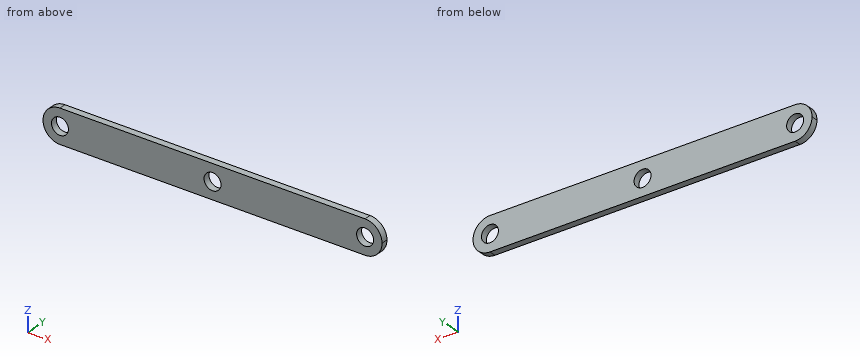
```python
from build123d import *

# Parameters (mm, degrees)
F0_W     = 100
F0_H     = 10
F0_R     = 2.5
F1_DEPTH = 2
F2_R     = 4.99999


# Not quite as in the source:
# - a fillet or chamfer is up to 0.001 mm smaller than in the source, because OpenCascade refuses the exact size


with BuildPart() as f1:
    # F0 (on Front) → F1 (new body)
    with BuildSketch(Plane.XZ):
        Rectangle(F0_W, F0_H)
        with Locations((-45, 0)):
            Circle(F0_R, mode=Mode.SUBTRACT)
        Circle(F0_R, mode=Mode.SUBTRACT)
        with Locations((45, 0)):
            Circle(F0_R, mode=Mode.SUBTRACT)
    extrude(amount=F1_DEPTH)

    # F2 (radius 5 in the source; OpenCascade refuses exactly that, so slightly less here)
    f2_edges = [f1.edges().sort_by_distance(p)[0] for p in [
        (-50, -1, 5),
        (-50, -1, -5),
        (50, -1, -5),
        (50, -1, 5),
    ]]
    fillet(f2_edges, radius=F2_R)


with BuildPart() as f3_1:
    # F3: copy of F1
    add(f1.part.moved(Location((0, -2, 0))))


solid = f1.part
```
Geometry: final body of the model. Coordinates: model frame, mm. Coordinates: 2 decimals unless noted, no trailing zeros. Order: outer loops, then holes, each group sorted by start corner. A loop starts at its lowest first (then second) coordinate and runs counter-clockwise, first axis right, second up. Notation, with made-up numbers: M 89,69.25 L 130,69.25 A27 ccw 130,95.25 Z; hole C 23.5,-3 d6. An arc over 180 degrees is marked long. Answer in a Markdown table with one row per item. Add a question column.
Q1. Section query B-B on x = 0. Return the cut outline in (y, z).
Q2. Section query C-C on z = 1.5. Return the cut outline in (x, y), and give its area (3 significant figures).
Q3. Line query: L1, parallel to Z at x = 45, y = -0.65; L2, parallel to X at y = -0.4, z = -2; L3, parallel to X at y = -0.45, z = 1.5. Output: solid intervals per line, ascending.
Q4. Section query A-A on y = -0.95. Count the separate pieces of the cut face and the enclosed holes in it, and give its area (3 significant figures).
Q5. Contact query for a flat-ended pin moving along its axis: P1, Ø4.5, axis at x = -45, z = 0, coming from the +Y side. Output: stop coordinate, or through.
Completed:
| question | item | result |
|---|---|---|
| 1 | outline | M -2,-5 L 0,-5 L 0,-2.5 L -2,-2.5 Z; M -2,2.5 L 0,2.5 L 0,5 L -2,5 Z |
| 2 | outline | M -49.77,-2 L -47,-2 L -47,0 L -49.77,0 Z; M -43,-2 L -2,-2 L -2,0 L -43,0 Z; M 2,-2 L 43,-2 L 43,0 L 2,0 Z; M 47,-2 L 49.77,-2 L 49.77,0 L 47,0 Z |
| 2 | area | 175 mm2 |
| 3 | L1 | z = -5 to -2.5, 2.5 to 5 |
| 3 | L2 | x = -49.58 to -46.5, -43.5 to -1.5, 1.5 to 43.5, 46.5 to 49.58 |
| 3 | L3 | x = -49.77 to -47, -43 to -2, 2 to 43, 47 to 49.77 |
| 4 | separate pieces | 1 |
| 4 | enclosed holes | 3 |
| 4 | area | 920 mm2 |
| 5 | P1 | passes through |
